Can you work these out from the model? Positions are in its coordinate system, mm. A direction names the side the tool comes from. Give positions to 0.01 mm unless a question says otherwise; leave off trailing zeros. Write each loop counter-clockwise with the first axis right and the second up, starting at its lowest first coordinate (ties: lowest second). Pieces come first, ordered by that corner, then holes.
```python
from build123d import *

# Parameters (mm, degrees)
PAD014_DEPTH           = 5
CYLINDER018_R          = 10
CYLINDER018_DEPTH      = 68.5
CYLINDER018_ROLL_ANGLE = 90
CYLINDER001_R          = 2.4
CYLINDER001_DEPTH      = 200
CYLINDER001_ROLL_ANGLE = 90
CYLINDER017_R          = 20
CYLINDER017_DEPTH      = 73
CYLINDER017_ROLL_ANGLE = 90
CYLINDER_R             = 50
CYLINDER_DEPTH         = 70
CYLINDER_ROLL_ANGLE    = 90
TORUS_R                = 35
TORUS_ROLL_ANGLE       = 90


with BuildPart() as pad014:
    # Sketch011 → Pad014 (new body)
    with BuildSketch(Plane.XZ.offset(36.5)):
        Polygon((4.618802, 0), (2.309401, 4), (-2.309401, 4), (-4.618802, 0), (-2.309401, -4), (2.309401, -4), align=None)
    extrude(amount=-PAD014_DEPTH)


with BuildPart() as cilindro018:
    # Cylinder018 → Cylinder018 (new body)
    with BuildSketch(Plane.XY):
        Circle(CYLINDER018_R)
    extrude(amount=CYLINDER018_DEPTH)


with BuildPart() as cilindro018_1:
    # Cylinder018 roll: moved
    add(cilindro018.part.rotate(Axis((0, 0, 0), (1, 0, 0)), CYLINDER018_ROLL_ANGLE))


with BuildPart() as cilindro018_2:
    # Cylinder018 placement: moved
    add(cilindro018_1.part.moved(Location((0, 100, 0))))


with BuildPart() as cilindro001:
    # Cylinder001 → Cylinder001 (new body)
    with BuildSketch(Plane.XY):
        Circle(CYLINDER001_R)
    extrude(amount=CYLINDER001_DEPTH)


with BuildPart() as cilindro001_1:
    # Cylinder001 roll: moved
    add(cilindro001.part.rotate(Axis((0, 0, 0), (1, 0, 0)), CYLINDER001_ROLL_ANGLE))


with BuildPart() as cilindro001_2:
    # Cylinder001 placement: moved
    add(cilindro001_1.part.moved(Location((0, 100, 0))))


with BuildPart() as cilindro017:
    # Cylinder017 → Cylinder017 (new body)
    with BuildSketch(Plane.XY):
        Circle(CYLINDER017_R)
    extrude(amount=CYLINDER017_DEPTH)


with BuildPart() as cilindro017_1:
    # Cylinder017 roll: moved
    add(cilindro017.part.rotate(Axis((0, 0, 0), (1, 0, 0)), CYLINDER017_ROLL_ANGLE))


with BuildPart() as cilindro017_2:
    # Cylinder017 placement: moved
    add(cilindro017_1.part.moved(Location((0, 36.5, 0))))


with BuildPart() as cilindro:
    # Cylinder → Cylinder (new body)
    with BuildSketch(Plane.XY):
        Circle(CYLINDER_R)
    extrude(amount=CYLINDER_DEPTH)


with BuildPart() as cilindro_1:
    # Cylinder roll: moved
    add(cilindro.part.rotate(Axis((0, 0, 0), (1, 0, 0)), CYLINDER_ROLL_ANGLE))


with BuildPart() as cilindro_2:
    # Cylinder placement: moved
    add(cilindro_1.part.moved(Location((0, 35, 0))))


with BuildPart() as cut017:
    # Torus → Torus (revolve)
    with BuildSketch(Plane.XZ):
        with Locations((50, 0)):
            Circle(TORUS_R)
    revolve(axis=Axis((0, 0, 0), (0, 0, 1)))


with BuildPart() as cut017_1:
    # Torus roll: moved
    add(cut017.part.rotate(Axis((0, 0, 0), (1, 0, 0)), TORUS_ROLL_ANGLE))


with BuildPart() as cut017_2:
    # Torus placement: moved
    add(cut017_1.part)

    # Fusion: union Cilindro
    add(cilindro_2.part)

    # Fusion016: union Cilindro017
    add(cilindro017_2.part)

    # Cut011: cut Cilindro001
    add(cilindro001_2.part, mode=Mode.SUBTRACT)

    # Cut012: cut Cilindro018
    add(cilindro018_2.part, mode=Mode.SUBTRACT)

    # Cut017: cut Pad014
    add(pad014.part, mode=Mode.SUBTRACT)


solid = cut017_2.part
```
1) Suppose I cut it at B-B on y = 18.5. Write out the boundary of the cut face in (x, z), plus the area to 3 significant figures.
Values follow:
outline: circle Ø159.42 at (0, 0); hole circle Ø4.8 at (0, 0)
area: 19,900 mm2
2) Suppose I cut it at A-A on x = 0. Write out the boundary of the cut face in (y, z), plus the area to 3 significant figures.
Values follow:
outline: (-36.5, -20) - (-35, -20) - (-35, -50) arc R35 ccw to (35, -50) - (35, -20) - (36.5, -20) - (36.5, -10) - (31.5, -10) - (31.5, -2.4) - (-31.5, -2.4) - (-31.5, -4) - (-36.5, -4) - close; (-36.5, 4) - (-31.5, 4) - (-31.5, 2.4) - (31.5, 2.4) - (31.5, 10) - (36.5, 10) - (36.5, 20) - (35, 20) - (35, 50) arc R35 ccw to (-35, 50) - (-35, 20) - (-36.5, 20) - close
area: 10,500 mm2
3) For pin 1 Ø4 at (x, z) = (-29.5, -33.5) entering from -Y; pin 2 Ø6.5 at (x, z) = (1.5, 2) entering from -Y; pin 3 Ø5 at (x, y) = (48.5, -14) entering from -Z; pin 4 Ø12 at (x, z) = (45.5, 3.5) entering from +Y, each with a flat end and sliding along its axis, tell me the tip position at first contact or that it passes through.
Values follow:
pin 1: stops at y = -35
pin 2: stops at y = -36.5
pin 3: stops at z = -68.38
pin 4: stops at y = 35
4) Suppose I cut it at C-C on y = -14. Write out the boundary of the cut face in (x, z), plus the area to 3 significant figures.
Values follow:
outline: circle Ø164.16 at (0, 0); hole circle Ø4.8 at (0, 0)
area: 21,100 mm2
5) Please list where these lines run through material, in increasing order: L1, parallel to Z at x = 0, y = 11; L2, parallel to Z at x = 0, y = -18; L3, parallel to Y at x = -21.5, z = -7.5.
Values follow:
L1: z = -83.23 to -2.4, 2.4 to 83.23
L2: z = -80.02 to -2.4, 2.4 to 80.02
L3: y = -35 to 35
6) For faces 1 (the face through (-1, 35, -22)), 2 (the face through (-5, 36.5, 9)), 3 (the face through (2, -31.5, 2)), which set-ups out of +Z, -Z, +X, -X, +Y, -Y let a thin tool reach every point of the face, with its end or its side?
Values follow:
face 1: +Y
face 2: +Z, -Z, +X, -X, +Y
face 3: -Y
7) If we mould it in two halves opening along X, with no side actions, what happens to faces 4 (the face through (-4.336, 35.76, -19.524)), 5 (the face through (-1, -35, -22)), 6 (the face through (2, 31.5, -2))? For each: +X half, -X half, draft (parallel to the pull), parting line (faces both ways), or undercut.
Values follow:
face 4: parting line
face 5: draft
face 6: undercut
